from build123d import *

# Parameters (mm, degrees)
BOSS_EXTRUDE1_DEPTH                                  = 3
CSK_FOR_M1_6_COUNTERSUNK_FLAT_HEAD_SCREW_D           = 1.7
CSK_FOR_M1_6_COUNTERSUNK_FLAT_HEAD_SCREW_CSINK_D     = 2
CSK_FOR_M1_6_COUNTERSUNK_FLAT_HEAD_SCREW_CSINK_ANGLE = 90


with BuildPart() as part:
    # Sketch1 → Boss-Extrude1 (new body)
    with BuildSketch(Plane.XY):
        with BuildLine():
            Line((8.75, -3.75), (4.75, -3.75))
            Line((4.75, -3.75), (4.75, -2.75))
            ThreePointArc((4.75, -2.75), (4.164213562, -1.335786438), (2.75, -0.75))
            Line((2.75, -0.75), (-2.75, -0.75))
            ThreePointArc((-2.75, -0.75), (-4.164213562, -1.335786438), (-4.75, -2.75))
            Line((-4.75, -2.75), (-4.75, -3.75))
            Line((-4.75, -3.75), (-8.75, -3.75))
            Line((-8.75, -3.75), (-8.75, 1.25))
            ThreePointArc((-8.75, 1.25), (-8.017766953, 3.017766953), (-6.25, 3.75))
            Line((-6.25, 3.75), (-2.2, 3.75))
            ThreePointArc((-2.2, 3.75), (-1.528248558, 3.471751442), (-1.25, 2.8))
            ThreePointArc((-1.25, 2.8), (0, 1.55), (1.25, 2.8))
            ThreePointArc((1.25, 2.8), (1.528248558, 3.471751442), (2.2, 3.75))
            Line((2.2, 3.75), (6.25, 3.75))
            ThreePointArc((6.25, 3.75), (8.017766953, 3.017766953), (8.75, 1.25))
            Line((8.75, 1.25), (8.75, -3.75))
        make_face()
    extrude(amount=BOSS_EXTRUDE1_DEPTH)

    # CSK for M1.6 Countersunk Flat Head Screw1 (through all)
    with Locations(Plane(origin=(0, -3.75, 0), x_dir=(-1, 0, 0), z_dir=(0, -1, 0))):
        with Locations((6.75, -1.5), (-6.75, -1.5)):
            CounterSinkHole(CSK_FOR_M1_6_COUNTERSUNK_FLAT_HEAD_SCREW_D / 2, CSK_FOR_M1_6_COUNTERSUNK_FLAT_HEAD_SCREW_CSINK_D / 2, counter_sink_angle=CSK_FOR_M1_6_COUNTERSUNK_FLAT_HEAD_SCREW_CSINK_ANGLE)


solid = part.part
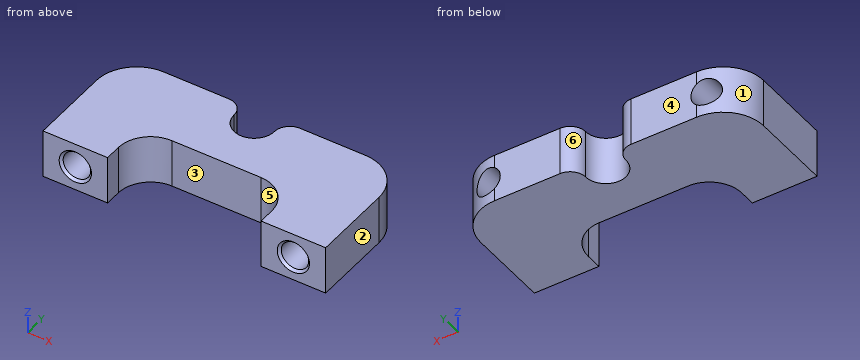
Source: CAD feature listing. Evaluate the final solid. Frame: model axes, mm. Face numbers are marked on the shaded views. A direction names the side the tool comes from. Coordinates: 2 decimals unless noted, no trailing zeros. Write each loop counter-clockwise with the first axis right and the second up, starting at its lowest first coordinate (ties: lowest second). Pieces come first, ordered by that corner, then holes. Notation, with made-up numbers: M 16,-4.5 L 25,-4.5 A32 ccw 25,30.5 Z; hole C 24,42.5 d6. An arc over 180 degrees is marked long. Use a Markdown table: item, result.
1) Section C-C, the plane x = -6.75. Output: boundary loops of the cut face in (y, z), then the cut area to 3 significant figures.
Conclusion:
| item | result |
|---|---|
| outline | M -3.75,0 L 3.7,0 L 3.7,0.65 L -3.6,0.65 L -3.75,0.5 Z; M -3.75,2.5 L -3.6,2.35 L 3.7,2.35 L 3.7,3 L -3.75,3 Z |
| area | 9.66 mm^2 |
2) Ray query, L1, parallel to X at y = -2, z = 1.9; L2, parallel to X at y = 1.25, z = 1.9; L3, parallel to X at y = -1.5, z = 0.85. Return the intervals inside material, ascending.
Conclusion:
| item | result |
|---|---|
| L1 | x = -8.75 to -7.5, -6 to -4.6, 4.6 to 6, 7.5 to 8.75 |
| L2 | x = -8.75 to -7.5, -6 to 6, 7.5 to 8.75 |
| L3 | x = -8.75 to -7.3, -6.2 to -4.31, 4.31 to 6.2, 7.3 to 8.75 |
3) Mould query, pull axis X, two halves, no side actions, for the marked faces 1, 2 and 3. Classes: pulls with the +X half, pulls with the -X half, needs draft (parallel to the pull), parting line crosses it, or undercut.
Conclusion:
| item | result |
|---|---|
| face 1 | pulls with the -X half |
| face 2 | pulls with the +X half |
| face 3 | undercut |
4) First-contact query: pin 1 Ø1.5 at (x, z) = (0.5, 1.5) entering from -Y. Flat tip, straight axial feed; report the tip coordinate or a pass-through.
Conclusion:
| item | result |
|---|---|
| pin 1 | stops at y = -0.75 |
5) Section D-D, the plane y = -0.25. Output: boundary loops of the cut face in (x, z).
Conclusion:
| item | result |
|---|---|
| outline | M -8.75,0 L 8.75,0 L 8.75,3 L -8.75,3 Z; hole C -6.75,1.5 d1.7; hole C 6.75,1.5 d1.7 |
6) Section B-B, the plane y = -2. Output: boundary loops of the cut face in (x, z).
Conclusion:
| item | result |
|---|---|
| outline | M -8.75,0 L -4.6,0 L -4.6,3 L -8.75,3 Z; M 4.6,0 L 8.75,0 L 8.75,3 L 4.6,3 Z; hole C -6.75,1.5 d1.7; hole C 6.75,1.5 d1.7 |
7) Reachability of the marked faces 4, 5 and 6 from +Z, -Z, +X, -X, +Y, -Y: full face, straight path, thin tool, end or side. Return the list, or none.
Conclusion:
| item | result |
|---|---|
| face 4 | +Z, -Z, +X, -X, +Y |
| face 5 | +Z, -Z, -Y |
| face 6 | +Z, -Z, +Y |
8) Section A-A, the plane z = 1.5. Output: boundary loops of the cut face in (x, y).
Conclusion:
| item | result |
|---|---|
| outline | M -8.75,-3.75 L -7.75,-3.75 L -7.6,-3.6 L -7.6,3.35 A2.5 ccw -8.75,1.25 Z; M -5.9,-3.6 L -5.75,-3.75 L -4.75,-3.75 L -4.75,-2.75 A2 cw -2.75,-0.75 L 2.75,-0.75 A2 cw 4.75,-2.75 L 4.75,-3.75 L 5.75,-3.75 L 5.9,-3.6 L 5.9,3.75 L 2.2,3.75 A0.95 ccw 1.25,2.8 A1.25 cw -1.25,2.8 A0.95 ccw -2.2,3.75 L -5.9,3.75 Z; M 7.6,-3.6 L 7.75,-3.75 L 8.75,-3.75 L 8.75,1.25 A2.5 ccw 7.6,3.35 Z |
